from build123d import *

# Parameters (mm, degrees)
SKETCH1_R           = 10
BOSS_EXTRUDE2_DEPTH = 6


with BuildPart() as part:
    # Sketch1 → Boss-Extrude2 (new body)
    with BuildSketch(Plane.XY):
        Polygon((-35, 51), (-45, 51), (-45, 45), (-50, 45), (-55, 40), (-55, -40), (-50, -45), (-45, -45), (-45, -51), (-35, -51), (-35, -45), (35, -45), (35, -51), (45, -51), (45, -45), (50, -45), (55, -40), (55, 40), (50, 45), (45, 45), (45, 51), (35, 51), (35, 45), (-35, 45), align=None)
        Polygon((33.096829988, 36), (35.596829988, 33.5), (20.596829988, 33.5), (23.096829988, 36), align=None, mode=Mode.SUBTRACT)
        with BuildLine():
            ThreePointArc((31.096829988, 0), (0, -31.096829988), (-31.096829988, 0))
            ThreePointArc((-31.096829988, 0), (-28.096829988, 3), (-25.096829988, 0))
            ThreePointArc((-25.096829988, 0), (0, -25.096829988), (25.096829988, 0))
            ThreePointArc((25.096829988, 0), (28.096829988, 3), (31.096829988, 0))
        make_face(mode=Mode.SUBTRACT)
        with Locations((-28.096829988, 20)):
            Circle(SKETCH1_R, mode=Mode.SUBTRACT)
        Polygon((-35.596829988, 33.5), (-33.096829988, 36), (-23.096829988, 36), (-20.596829988, 33.5), align=None, mode=Mode.SUBTRACT)
        with Locations((28.096829988, 20)):
            Circle(SKETCH1_R, mode=Mode.SUBTRACT)
    extrude(amount=BOSS_EXTRUDE2_DEPTH)


solid = part.part
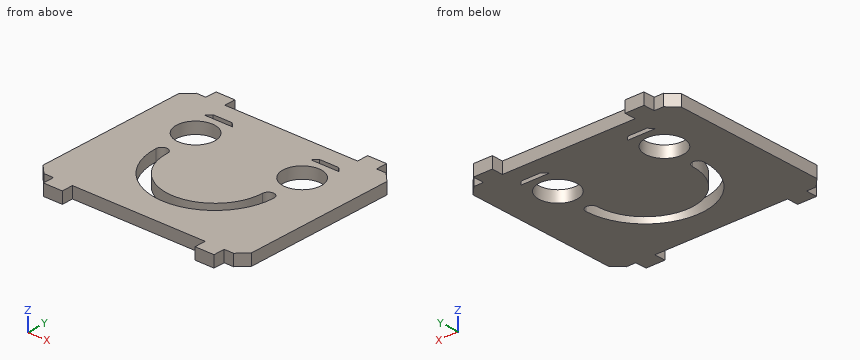
Build history of the part. All positions in model axes, mm. Round coordinates to 2 decimals unless told otherwise and drop trailing zeros. Write each loop counter-clockwise with the first axis right and the second up, starting at its lowest first coordinate (ties: lowest second). Pieces come first, ordered by that corner, then holes. Notation, with made-up numbers: M -29.5,67.5 L 3.5,67.5 A25 ccw 3.5,96.5 Z; hole C 57.5,-39 d7. An arc over 180 degrees is marked long. Use CSV: the item, a comma, the result in double quotes.
1. Saw through at B-B (x = 0). Give the cut face in (y, z).
Reply:
outline,"M -45,0 L -31.1,0 L -31.1,6 L -45,6 Z; M -25.1,0 L 45,0 L 45,6 L -25.1,6 Z"
2. Flat gauge pins, fed straight in: pin 1 (3 mm diameter, centred on x = -24.5, z = 4.5, fed in from +Y); pin 2 (3 mm diameter, centred on y = 48.5, z = 3.5, fed in from -X); pin 3 (3 mm diameter, centred on x = 26, z = 2, fed in from -Y); pin 4 (16 mm diameter, centred on x = 28.1, y = 20, fed in from -Z). Where does each tip first touch, or does it go through?
Reply:
pin 1,"stops at y = 45"
pin 2,"stops at x = -45"
pin 3,"stops at y = -45"
pin 4,"passes through"
3. Wall check: probe 1 along X at (y, z) = (46, 1.4); probe 2 along X at (y, z) = (-15, 1.85); probe 3 along X at (y, z) = (-13.5, 5.1). Give the ranges that are in metal, low to high. Write a range as from..to.
Reply:
probe 1,"x = -45..-35, 35..45"
probe 2,"x = -55..-27.24, -20.12..20.12, 27.24..55"
probe 3,"x = -55..-28.01, -21.16..21.16, 28.01..55"
4. Saw through at D-D (y = -6). Give the cut face in (x, z), plus the area to 3 significant figures.
Reply:
outline,"M -55,0 L -30.51,0 L -30.51,6 L -55,6 Z; M -24.37,0 L 24.37,0 L 24.37,6 L -24.37,6 Z; M 30.51,0 L 55,0 L 55,6 L 30.51,6 Z"
area,"586 mm²"
5. Saw through at A-A (y = 20). Give the cut face in (x, z).
Reply:
outline,"M -55,0 L -38.1,0 L -38.1,6 L -55,6 Z; M -18.1,0 L 18.1,0 L 18.1,6 L -18.1,6 Z; M 38.1,0 L 55,0 L 55,6 L 38.1,6 Z"
6. Saw through at C-C (z = 1.2). State how many separate pieces and enclosed holes the cut face has, plus the area to 3 significant figures.
Reply:
separate pieces,"1"
enclosed holes,"5"
area,"8,840 mm²"
